The model under review builds one solid part; all positions refer to its coordinate system, in mm. A direction names the side the tool comes from. Give positions to 0.01 mm unless a question says otherwise; leave off trailing zeros. Order: outer loops, then holes, each group sorted by start corner. A loop starts at its lowest first (then second) coordinate and runs counter-clockwise, first axis right, second up. Notation, with made-up numbers: (5, 23) - (16, 23) arc R16 ccw to (16, 50) - close; hole circle Ø6 at (74.5, -10). An arc over 180 degrees is marked (long way). Write item = value, one per line. Start each with the question number.
1. Machinability: for faces 1 (the flat face through (0, 11, 0)), 2 (the flat face through (0, -5.5, 2)), 3 (the flat face through (-9, 31, 8)), 4 (the flat face through (15, 13, 2)), which of the approach directions +Z, -Z, +X, -X, +Y, -Y give a long, thin tool a straight path to every point of the face, cutting with its end or side? Answer none if there is none.
2. We need section A-A, the plane y = -3.5. Give the boundary of the cut face in (x, z), and give its area (3 significant figures).
3. We need section D-D, the plane x = -13. Give the boundary of the cut face in (y, z), and give its area (3 significant figures).
4. For P1, Ø1.5, axis at y = 17.5, z = 2, coming from the +X side; P2, Ø4, axis at x = 7.5, z = 11.5, coming from the -Y side; P3, Ø12, axis at x = 15, y = 28, coming from the -Z side; P4, Ø1, axis at y = 12.5, z = 2.5, coming from the -X side, all flat-tipped, find the tip position at first contact; note any pin that passes through.
5. We need section B-B, the plane x = -3. Give the boundary of the cut face in (y, z), and give its area (3 significant figures).
6. Wall thickness on probe 1 along X at (y, z) = (1, 1.75); probe 2 along Y at (x, z) = (-9.75, 2); probe 3 along X at (y, z) = (31.9, 10): over which ranges is each line inside the solid? List them lowest first.
7. Mouldability with a two-part tool opening along X and no side actions: class faces 5 (the cylindrical face through (8.1, 31.48, 3.86)), 6 (the cylindrical face through (-13, -9, 2)), 7 (the flat face through (0, -10, 2)), 8 (the cylindrical face through (-9.9, 31.48, 12.14)) as pulls with the +X half, pulls with the -X half, needs draft (parallel to the pull), parting line crosses it, or undercut.
8. We need section C-C, the plane y = 28.5. Give the boundary of the cut face in (x, z), and give its area (3 significant figures).
from build123d import *
from build123d.topology import SkipClean

# Parameters (mm, degrees)
SKETCH1_W           = 25
SKETCH1_H           = 20
SKETCH1_R           = 1.5
BOSS_EXTRUDE1_DEPTH = 3
SKETCH2_W           = 15.54
SKETCH2_H           = 11
CUT_EXTRUDE1_DEPTH  = 17.286497475
SKETCH4_W           = 25
SKETCH4_H           = 3
BOSS_EXTRUDE2_DEPTH = 3
SKETCH5_W           = 25
SKETCH5_H           = 3
BOSS_EXTRUDE3_DEPTH = 10
SKETCH11_W          = 25
SKETCH11_H          = 13
BOSS_EXTRUDE5_DEPTH = 20
SKETCH12_W          = 25
SKETCH12_H          = 10
CUT_EXTRUDE4_DEPTH  = 20
BOSS_EXTRUDE6_DEPTH = 2.5
BOSS_EXTRUDE7_DEPTH = 2.5
SKETCH16_R          = 1.75
CUT_EXTRUDE5_DEPTH  = 45.654227124
FILLET6_R           = 3
FILLET7_R           = 3
CUT_EXTRUDE6_DEPTH  = 45.654227124
FILLET8_R           = 5
BOSS_EXTRUDE8_DEPTH = 3


with BuildPart() as part:
    # Sketch1 → Boss-Extrude1 (new body)
    with BuildSketch(Plane.XY):
        Rectangle(SKETCH1_W, SKETCH1_H)
        with Locations((-9.75, 0)):
            Circle(SKETCH1_R, mode=Mode.SUBTRACT)
        with Locations((9.75, 0)):
            Circle(SKETCH1_R, mode=Mode.SUBTRACT)
    extrude(amount=BOSS_EXTRUDE1_DEPTH)

    # Sketch2 → Cut-Extrude1 (cut, through all)
    with BuildSketch(Plane.XY.offset(3)):
        Rectangle(SKETCH2_W, SKETCH2_H)
    extrude(amount=-CUT_EXTRUDE1_DEPTH, mode=Mode.SUBTRACT)

    # Sketch4 → Boss-Extrude2 (add)
    with BuildSketch(Plane(origin=(0, 10, 0), x_dir=(1, 0, 0), z_dir=(0, 1, 0))):
        with Locations((0, -1.5)):
            Rectangle(SKETCH4_W, SKETCH4_H)
    extrude(amount=BOSS_EXTRUDE2_DEPTH)

    # Sketch5 → Boss-Extrude3 (add)
    with BuildSketch(Plane.XY.offset(3)):
        with Locations((0, 11.5)):
            Rectangle(SKETCH5_W, SKETCH5_H)
    extrude(amount=BOSS_EXTRUDE3_DEPTH)

    # Sketch11 → Boss-Extrude5 (add)
    with BuildSketch(Plane(origin=(0, 13, 0), x_dir=(1, 0, 0), z_dir=(0, 1, 0))):
        with Locations((0, -6.5)):
            Rectangle(SKETCH11_W, SKETCH11_H)
    extrude(amount=BOSS_EXTRUDE5_DEPTH)

    # Sketch12 → Cut-Extrude4 (cut)
    with BuildSketch(Plane.XZ.offset(-10)):
        with Locations((0, 8)):
            Rectangle(SKETCH12_W, SKETCH12_H)
    extrude(amount=-CUT_EXTRUDE4_DEPTH, mode=Mode.SUBTRACT)

    # Sketch13 → Boss-Extrude6 (add)
    with BuildSketch(Plane.ZY.offset(12.5)):
        Polygon((3, -10), (3, 30), (13, 30), (13, 33), (0, 33), (0, -10), align=None)
    extrude(amount=BOSS_EXTRUDE6_DEPTH)

    # Sketch14 → Boss-Extrude7 (add)
    with BuildSketch(Plane(origin=(12.5, 0, 0), x_dir=(0, 0, -1), z_dir=(1, 0, 0))):
        Polygon((-13, 30), (-3, 30), (-3, -10), (0, -10), (0, 33), (-13, 33), align=None)
    extrude(amount=BOSS_EXTRUDE7_DEPTH)

    # Sketch16 → Cut-Extrude5 (cut, through all)
    with BuildSketch(Plane.XZ.offset(-30)):
        with Locations(Location((-12, 10, 0), (0, 0, 270))):
            Circle(SKETCH16_R)
        with Locations(Location((12, 10, 0), (0, 0, 270))):
            Circle(SKETCH16_R)
    extrude(amount=-CUT_EXTRUDE5_DEPTH, mode=Mode.SUBTRACT)

    # Fillet6
    fillet6_edges = [part.edges().sort_by_distance(p)[0] for p in [
        (-15, 31.5, 13),
    ]]
    fillet(fillet6_edges, radius=FILLET6_R)

    # Fillet7
    fillet7_edges = [part.edges().sort_by_distance(p)[0] for p in [
        (15, 31.5, 13),
    ]]
    fillet(fillet7_edges, radius=FILLET7_R)

    # Sketch17 → Cut-Extrude6 (cut, through all)
    with SkipClean():  # the faces are left unmerged after this step: merging them gives an invalid solid
        with BuildSketch(Plane.XZ.offset(-30)):
            with BuildLine():
                Line((-9, 10), (-9, 6))
                ThreePointArc((-9, 6), (-8.121320344, 3.878679656), (-6, 3))
                Line((-6, 3), (6, 3))
                ThreePointArc((6, 3), (8.121320344, 3.878679656), (9, 6))
                Line((9, 6), (9, 10))
                ThreePointArc((9, 10), (9.878679656, 12.121320344), (12, 13))
                Line((12, 13), (-12, 13))
                ThreePointArc((-12, 13), (-9.878679656, 12.121320344), (-9, 10))
            make_face()
        extrude(amount=-CUT_EXTRUDE6_DEPTH, mode=Mode.SUBTRACT)

    # Fillet8
    fillet8_edges = [part.edges().sort_by_distance(p)[0] for p in [
        (15, -10, 1.5),
        (-15, -10, 1.5),
    ]]
    fillet(fillet8_edges, radius=FILLET8_R)

    # Sketch18 → Boss-Extrude8 (add)
    with BuildSketch(Plane.XZ.offset(-30)):
        with BuildLine():
            Line((-12, 13), (-15.857475084, 13))
            Line((-15.857475084, 13), (-21.593636596, 4.395757731))
            Line((-21.593636596, 4.395757731), (-15, 0))
            Line((-15, 0), (-15, 10))
            ThreePointArc((-15, 10), (-14.121320344, 12.121320344), (-12, 13))
        make_face()
        with BuildLine():
            Line((12, 13), (15.857475084, 13))
            Line((15.857475084, 13), (21.593636596, 4.395757731))
            Line((21.593636596, 4.395757731), (15, 0))
            Line((15, 0), (15, 10))
            ThreePointArc((15, 10), (14.121320344, 12.121320344), (12, 13))
        make_face()
    extrude(amount=-BOSS_EXTRUDE8_DEPTH)


solid = part.part
Model answer:
q1.face_1 = -Z, +X, -X, +Y, -Y
q1.face_2 = +Z, -Z
q1.face_3 = +Z, +Y, -Y
q1.face_4 = +Z, -Z, +X, -Y
q2.outline = (-15, 0) - (-7.77, 0) - (-7.77, 3) - (-15, 3) - close; (7.77, 0) - (15, 0) - (15, 3) - (7.77, 3) - close
q2.area = 43.4 mm2
q3.outline = (-9, 0) - (33, 0) - (33, 8.56) - (30, 8.56) - (30, 3) - (-9, 3) - close; (30, 11.44) - (33, 11.44) - (33, 13) - (30, 13) - close
q3.area = 147 mm2
q4.P1 = 15
q4.P2 = 30
q4.P3 = 0
q4.P4 = -15
q5.outline = (-10, 0) - (-5.5, 0) - (-5.5, 3) - (-10, 3) - close; (5.5, 0) - (33, 0) - (33, 3) - (5.5, 3) - close
q5.area = 96.0 mm2
q6.probe_1 = -15 to -10.87, -8.63 to -7.77, 7.77 to 8.63, 10.87 to 15
q6.probe_2 = -10 to -1.5, 1.5 to 33
q6.probe_3 = -17.86 to -13.75, -10.25 to -9, 9 to 10.25, 13.75 to 17.86
q7.face_5 = undercut
q7.face_6 = pulls with the -X half
q7.face_7 = needs draft
q7.face_8 = undercut
q8.outline = (-15, 0) - (15, 0) - (15, 3) - (-15, 3) - close
q8.area = 90.0 mm2
